Part print with two shaded views. Sizes in mm from the minimum x, y, z corner. A direction names the side the tool comes from. Coordinates: 2 decimals unless noted, no trailing zeros. Loops run counter-clockwise (first coordinate to the right, second up) from the corner with the lowest first, then second, coordinate; pieces in that order, holes last. Notation, with made-up numbers: (-24, 45) -> (20, 45) arc R8 cw to (20, 50) -> close; hole circle Ø8 at (74, 83). An arc over 180 degrees is marked (long way). Return JSON: item names as keys, results as strings. Group by question number.
(1) Saw through at C-C on x = 2.25. Write the cut outline in (y, z) (1 decimal).
(2) Probe L1, parallel to X at y = 1.75, z = 2.5; L2, parallel to X at y = 1, z = 3 (1 decimal); L3, parallel to Z at x = 3, y = 5.5. List the from-to ranges inside material, lowest first.
(3) Saw through at D-D on y = 14.5. Write the cut outline in (x, z).
(4) Saw through at A-A on z = 1.3. Write the cut outline in (x, y) (1 decimal).
(5) Flat gauge pins, fed straight in: pin 1 Ø1.2 at (y, z) = (9, 1) entering from -X (1 decimal); pin 2 Ø2.5 at (y, z) = (9, 1) entering from +X. Where does each tip first touch, or does it go through?
(6) Tool access for the marked faces 1 and 2: list every direction of +Z, -Z, +X, -X, +Y, -Y with a clear straight run to the whole face (end or side of a thin tool).
(7) Saw through at B-B on z = 4.3. Write the cut outline in (x, y).
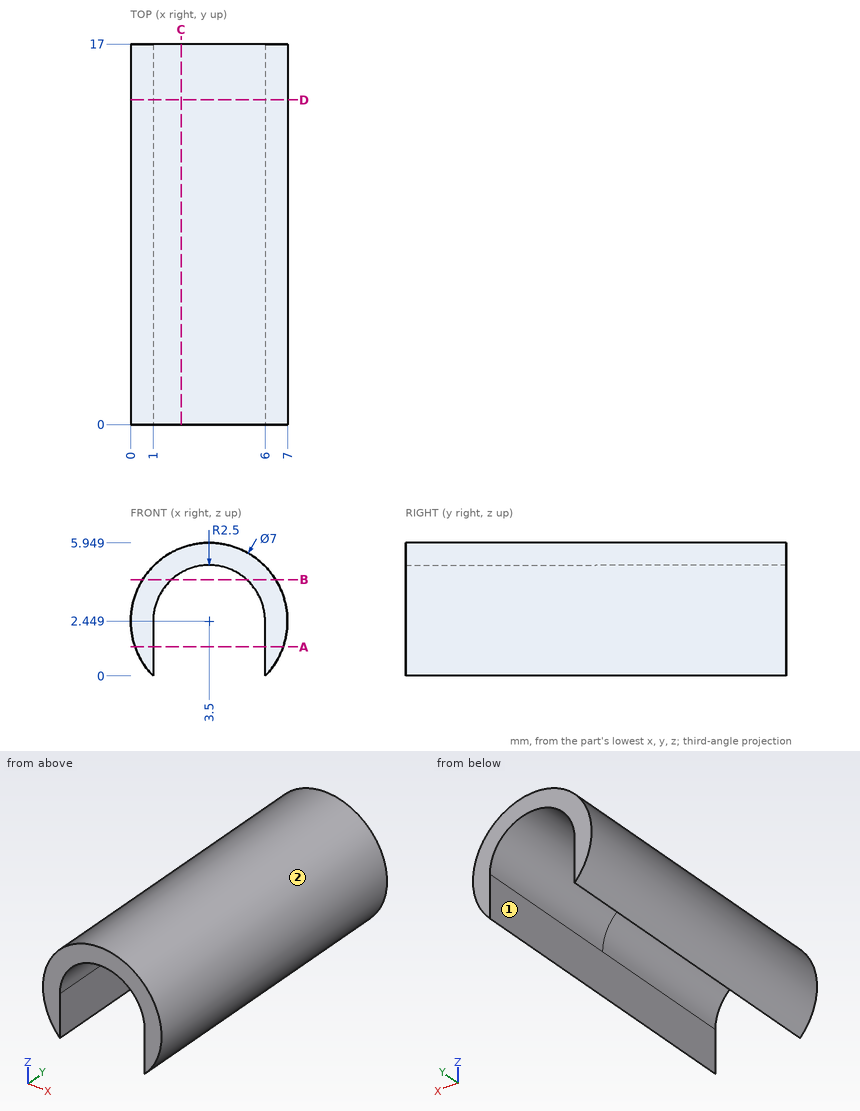
Geometry results:
{
 "1": {"outline": "(0, 4.6) -> (17, 4.6) -> (17, 5.7) -> (0, 5.7) -> close"},
 "2": {"L1": "0 to 1, 6 to 7", "L2": "0 to 1.1, 5.9 to 7", "L3": "4.9 to 5.91"},
 "3": {"outline": "(1, 0) -> (1, 2.45) arc R2.5 cw to (6, 2.45) -> (6, 0) arc R3.5 ccw (long way) to start"},
 "4": {"outline": "(0.2, 0) -> (1, 0) -> (1, 17) -> (0.2, 17) -> close; (6, 0) -> (6.8, 0) -> (6.8, 17) -> (6, 17) -> close"},
 "5": {"pin 1": "x = 0.1", "pin 2": "x = 6.99"},
 "6": {"face 1": "-Z, +Y, -Y", "face 2": "+Y, -Y"},
 "7": {"outline": "(0.53, 0) -> (1.82, 0) -> (1.82, 17) -> (0.53, 17) -> close; (5.18, 0) -> (6.47, 0) -> (6.47, 17) -> (5.18, 17) -> close"}
}
